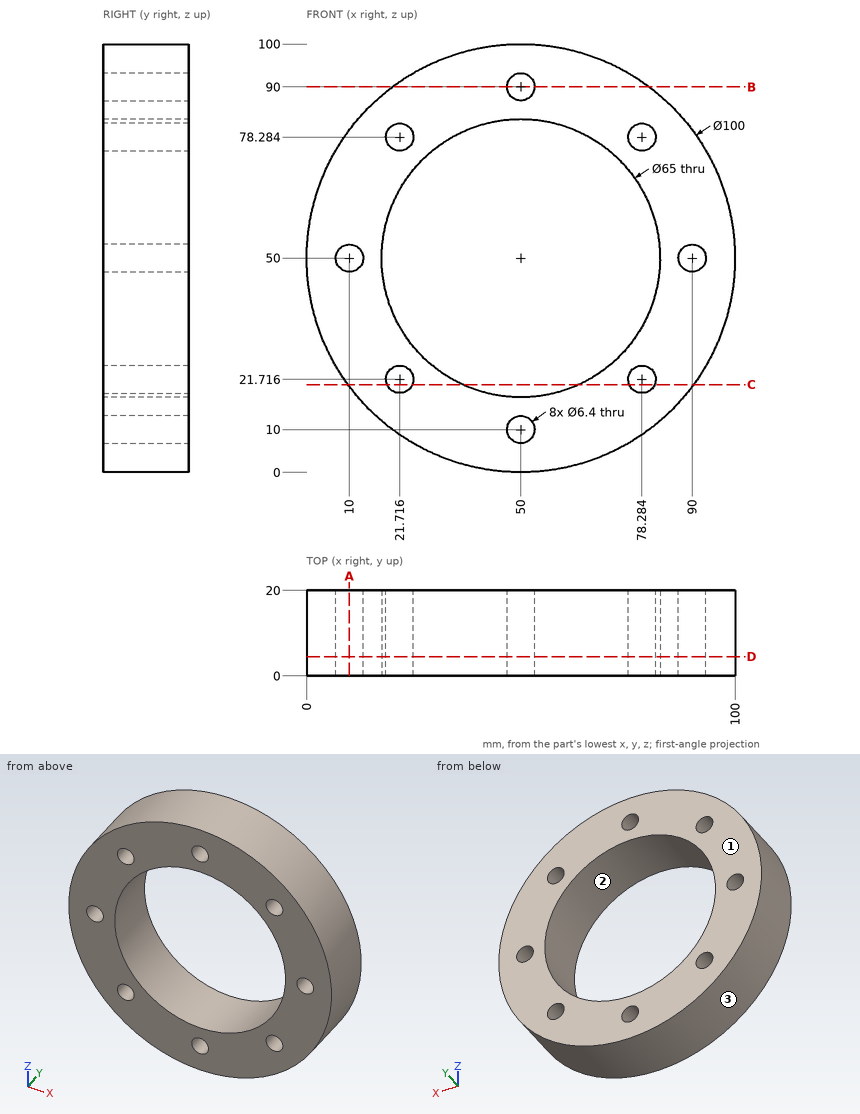
Design review of the part shown in the three views and the two pictorial views. Dimensions are in mm from the part's minimum x, y and z. Round coordinates to 2 decimals unless told otherwise and drop trailing zeros. Loops run counter-clockwise (first coordinate to the right, second up) from the corner with the lowest first, then second, coordinate; pieces in that order, holes last.
Q1. Add section A-A on x = 10. Write out the cut boundary in (y, z).
Result sheet:
outline: (0, 20) - (20, 20) - (20, 46.8) - (0, 46.8) - close; (0, 53.2) - (20, 53.2) - (20, 80) - (0, 80) - close
Q2. Add section D-D on y = 4.5. Give the number of separate pieces and of enclosed holes in the cut face, plus the area to 3 significant figures.
Result sheet:
separate pieces: 1
enclosed holes: 9
area: 4,280 mm2
Q3. Mouldability with a two-part tool opening along Z and no side actions: class the marked faces 1, 2 and 3 as +Z half, -Z half, draft (parallel to the pull), parting line (faces both ways), or undercut.
Result sheet:
face 1: draft
face 2: undercut
face 3: parting line
Q4. Add section B-B on z = 90. Write out the cut boundary in (x, y), plus the area to 3 significant figures.
Result sheet:
outline: (20, 0) - (46.8, 0) - (46.8, 20) - (20, 20) - close; (53.2, 0) - (80, 0) - (80, 20) - (53.2, 20) - close
area: 1,070 mm2
Q5. To check wall thickness, follow line 1 along X through (y, z) = (13.5, 50); line 2 along Z through (x, y) = (78.5, 10.75) (1 decimal); line 3 along Z through (x, y) = (76, 15) (1 decimal). State the ranges of each line that lie inside material, in increasing order.
Result sheet:
line 1: x = 0 to 6.8, 13.2 to 17.5, 82.5 to 86.8, 93.2 to 100
line 2: z = 8.9 to 18.5, 24.9 to 34.4, 65.6 to 75.1, 81.5 to 91.1
line 3: z = 7.3 to 19.5, 24 to 30.5, 69.5 to 76, 80.5 to 92.7
Q6. Insertion check: pin 1 Ø10 at (x, z) = (50, 10) entering from +Y; pin 2 Ø6 at (x, y) = (80.5, 17.5) entering from -Z; pin 3 Ø5 at (x, z) = (21.72, 21.72) entering from -Y; pin 4 Ø4 at (x, y) = (82.5, 6.5) entering from -Z. Each pin has a flat end and moves straight along its axis. Give the tip position at first contact, or say it passes through.
Result sheet:
pin 1: stops at y = 20
pin 2: stops at z = 8.24
pin 3: passes through
pin 4: stops at z = 10.38
Q7. Add section C-C on z = 20.5. Write out the cut boundary in (x, y).
Result sheet:
outline: (9.63, 0) - (18.76, 0) - (18.76, 20) - (9.63, 20) - close; (24.68, 0) - (36.36, 0) - (36.36, 20) - (24.68, 20) - close; (63.64, 0) - (75.32, 0) - (75.32, 20) - (63.64, 20) - close; (81.24, 0) - (90.37, 0) - (90.37, 20) - (81.24, 20) - close
